For this review, take the finished solid that the model builds, in its own axes (mm). Coordinates: 2 decimals unless noted, no trailing zeros. Write each loop counter-clockwise with the first axis right and the second up, starting at its lowest first coordinate (ties: lowest second). Pieces come first, ordered by that corner, then holes.
1) To check wall thickness, follow line 1 along Z through (x, y) = (4, 1.35); line 2 along Z through (x, y) = (2.75, 1.05); line 3 along X through (y, z) = (1.2, 6.5). State the ranges of each line that lie inside material, in increasing order.
2) We need section C-C on z = 5. Write out the cut boundary in (x, y), then the cut area to 3 significant figures.
3) We need section A-A on z = 17. Write out the cut boundary in (x, y), then the cut area to 3 significant figures.
4) Mouldability with a two-part tool opening along X and no side actions: class faces 1 (the face through (6.385, 0.986, 5.751)), 2 (the face through (0, 1, 25)), 3 (the face through (4, 2, 25)) as pulls with the +X half, pulls with the -X half, needs draft (parallel to the pull), parting line crosses it, or undercut.
5) We need section D-D on y = 1.6. Write out the cut boundary in (x, z), then the cut area to 3 significant figures.
6) We need section B-B on x = 2. Write out the cut boundary in (y, z).
Autodesk Inventor part; units mm, degrees
ref_plane "YZ Plane" through (0, 0, 0) normal (1, 0, 0) x (0, 1, 0)
ref_plane "XZ Plane" through (0, 0, 0) normal (0, 1, 0) x (-1, 0, 0)
ref_plane "XY Plane" through (0, 0, 0) normal (0, 0, 1) x (1, 0, 0)
sketch "Sketch1" plane through (0, 0, 0) normal (0, 0, 1) x (1, 0, 0)
  line L0 (0, 0) -> (8, 0)
  line L1 (8, 0) -> (8, 2)
  line L2 (8, 2) -> (0, 2)
  line L3 (0, 2) -> (0, 0)
  dimension "d0" = 8
  dimension "d1" = 2
extrude "Extrusion1" add sketch "Sketch1" along normal blind 50
sketch "Sketch2" plane through (0, 0, 0) normal (0, -1, 0) x (1, 0, 0)
  circle A0 centre (4, 5) radius 2.5
  circle A1 centre (4, 15) radius 2.5
  line L0 (0, 0) -> (8, 0)
  line L1 (8, 0) -> (8, 50)
  line L2 (0, 50) -> (8, 50)
  line L3 (0, 0) -> (0, 50)
  dimension "d4" = 5
  dimension "d5" = 5
  dimension "d6" = 5
  dimension "d7" = 10
  dimension "d8" = 4
  dimension "d9" = 4
extrude "Extrusion2" cut sketch "Sketch2" against normal up to next contours A0 | A1
properties part number "Y_Rail_Limit_Rod-SquareBar-Rev3"
Result:
1. line 1: z = 0 to 2.5, 7.5 to 12.5, 17.5 to 50
1. line 2: z = 0 to 2.83, 7.17 to 12.83, 17.17 to 50
1. line 3: x = 0 to 2, 6 to 8
2. outline: (0, 0) - (1.5, 0) - (1.5, 2) - (0, 2) - close; (6.5, 0) - (8, 0) - (8, 2) - (6.5, 2) - close
2. area: 6.00 mm2
3. outline: (0, 0) - (2.5, 0) - (2.5, 2) - (0, 2) - close; (5.5, 0) - (8, 0) - (8, 2) - (5.5, 2) - close
3. area: 10.0 mm2
4. face 1: undercut
4. face 2: pulls with the -X half
4. face 3: needs draft
5. outline: (0, 0) - (8, 0) - (8, 50) - (0, 50) - close; hole circle Ø5 at (4, 5); hole circle Ø5 at (4, 15)
5. area: 361 mm2
6. outline: (0, 0) - (2, 0) - (2, 3.5) - (0, 3.5) - close; (0, 6.5) - (2, 6.5) - (2, 13.5) - (0, 13.5) - close; (0, 16.5) - (2, 16.5) - (2, 50) - (0, 50) - close
